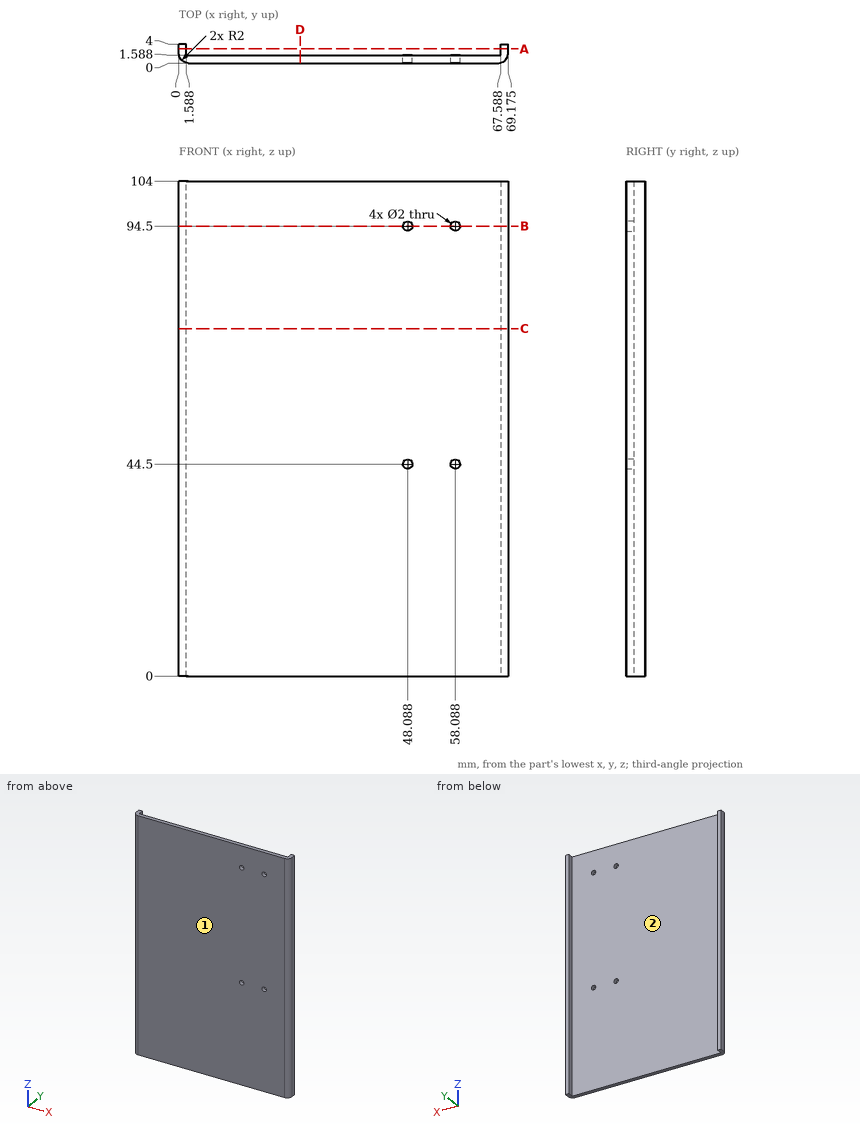
Source: three-view drawing plus pictorial views. Frame: mm from the lowest corner of the part. Round coordinates to 2 decimals unless told otherwise and drop trailing zeros. Write each loop counter-clockwise with the first axis right and the second up, starting at its lowest first coordinate (ties: lowest second). Pieces come first, ordered by that corner, then holes. Notation, with made-up numbers: M 39.5,-12 L 56.5,-12 A23 ccw 56.5,23 Z; hole C -2,44.5 d10. An arc over 180 degrees is marked long. Write item = value, one per line.
Item 1: Section query D-D on x = 25.5. Return loops of the section in (y, z), then the cut area to 3 significant figures.
Findings:
outline = M 0,0 L 1.59,0 L 1.59,104 L 0,104 Z
area = 165 mm^2
Item 2: Section query C-C on z = 73. Return loops of the section in (x, y) (1 decimal).
Findings:
outline = M 0,2 A2 ccw 2,0 L 67.2,0 A2 ccw 69.2,2 L 69.2,4 L 67.6,4 L 67.6,1.6 L 1.6,1.6 L 1.6,4 L 0,4 Z
Item 3: Pin query (flat end, axial travel): P1, Ø3, axis at x = 30.5, z = 23.5, coming from the +Y side. Return the tip coordinate at first contact, or that it passes through.
Findings:
P1 = 1.59
Item 4: Section query A-A on y = 2.95. Return loops of the section in (x, z) (1 decimal).
Findings:
outline = M 0,0 L 1.6,0 L 1.6,104 L 0,104 Z; M 67.6,0 L 69.2,0 L 69.2,104 L 67.6,104 Z
Item 5: Pull-direction query (X, two-part tool) for the marked faces 1 and 2; classes: pulls with the +X half, pulls with the -X half, needs draft (parallel to the pull), parting line crosses it, or undercut.
Findings:
face_1 = needs draft
face_2 = undercut
Item 6: Material intervals for line 1 along X through (y, z) = (3.55, 45) (1 decimal); line 2 along X through (y, z) = (1.1, 94.5) (1 decimal); line 3 along X through (y, z) = (0.95, 44.5) (1 decimal), sorted ascending. Write a range as [from, to].
Findings:
line_1 = [0, 1.6], [67.6, 69.2]
line_2 = [0.2, 47.1], [49.1, 57.1], [59.1, 69]
line_3 = [0.3, 47.1], [49.1, 57.1], [59.1, 68.9]
Item 7: Section query B-B on z = 94.5. Return loops of the section in (x, y) (1 decimal).
Findings:
outline = M 0,2 A2 ccw 2,0 L 47.1,0 L 47.1,1.6 L 1.6,1.6 L 1.6,4 L 0,4 Z; M 49.1,0 L 57.1,0 L 57.1,1.6 L 49.1,1.6 Z; M 59.1,0 L 67.2,0 A2 ccw 69.2,2 L 69.2,4 L 67.6,4 L 67.6,1.6 L 59.1,1.6 Z
